Part model, mm, in its own coordinate system. A direction names the side the tool comes from. Round coordinates to 2 decimals unless told otherwise and drop trailing zeros. Loops run counter-clockwise (first coordinate to the right, second up) from the corner with the lowest first, then second, coordinate; pieces in that order, holes last. Notation, with made-up numbers: (84.25, 44) -> (134.25, 44) arc R33 cw to (134.25, 78) -> close; hole circle Ø3 at (2, -37). An arc over 180 degrees is marked (long way). Answer as CSV lines item,"result".
from build123d import *

# Parameters (mm, degrees)
SKETCH1_W           = 39
SKETCH1_H           = 39
BOSS_EXTRUDE1_DEPTH = 29
SKETCH3_W           = 37
SKETCH3_H           = 27
CUT_EXTRUDE1_DEPTH  = 38
SKETCH4_W           = 35
SKETCH4_H           = 38.588060521
CUT_EXTRUDE2_DEPTH  = 10
CUT_EXTRUDE3_START  = 27
SKETCH5_W           = 40
SKETCH5_H           = 3
CUT_EXTRUDE3_DEPTH  = 4
CUT_EXTRUDE5_START  = 38
SKETCH6_W           = 41.777462506
SKETCH6_H           = 3
CUT_EXTRUDE5_DEPTH  = 1


with BuildPart() as part:
    # Sketch1 → Boss-Extrude1 (new body)
    with BuildSketch(Plane(origin=(0, 0, 0), x_dir=(1, 0, 0), z_dir=(0, 1, 0))):
        with Locations((-4.072718242, -0.197565543)):
            Rectangle(SKETCH1_W, SKETCH1_H)
    extrude(amount=BOSS_EXTRUDE1_DEPTH)

    # Sketch3 → Cut-Extrude1 (cut)
    with BuildSketch(Plane.XY.offset(19.697565543)):
        with Locations((-4.072718242, 14.5)):
            Rectangle(SKETCH3_W, SKETCH3_H)
    extrude(amount=-CUT_EXTRUDE1_DEPTH, mode=Mode.SUBTRACT)

    # Sketch4 → Cut-Extrude2 (cut)
    with BuildSketch(Plane(origin=(0, 29, 0), x_dir=(1, 0, 0), z_dir=(0, 1, 0))):
        with Locations((-4.072718242, -0.991595804)):
            Rectangle(SKETCH4_W, SKETCH4_H)
    extrude(amount=-CUT_EXTRUDE2_DEPTH, mode=Mode.SUBTRACT)

    # Sketch5 → Cut-Extrude3 (cut)
    with BuildSketch(Plane(origin=(0, 1, 0), x_dir=(1, 0, 0), z_dir=(0, 1, 0)).offset(CUT_EXTRUDE3_START)):
        with Locations((-4.288618926, -0.197565543)):
            Rectangle(SKETCH5_W, SKETCH5_H)
    extrude(amount=CUT_EXTRUDE3_DEPTH, mode=Mode.SUBTRACT)

    # Sketch6 → Cut-Extrude5 (cut)
    with BuildSketch(Plane.XY.offset(-18.302434457).offset(CUT_EXTRUDE5_START)):
        with Locations((-4.415990597, 14.5)):
            Rectangle(SKETCH6_W, SKETCH6_H)
    extrude(amount=-CUT_EXTRUDE5_DEPTH, mode=Mode.SUBTRACT)


solid = part.part
Q1. Saw through at A-A, the plane y = 20. Write the cut outline in (x, z), then the cut area to 3 significant figures.
Geometry results:
outline,"(-23.57, -19.3) -> (15.43, -19.3) -> (15.43, 19.7) -> (14.43, 19.7) -> (14.43, -18.3) -> (-22.57, -18.3) -> (-22.57, 19.7) -> (-23.57, 19.7) -> close"
area,"115 mm2"
Q2. Saw through at B-B, the plane x = 10.5. Write the cut outline in (y, z), then the cut area to 3 significant figures.
Geometry results:
outline,"(0, -19.3) -> (29, -19.3) -> (29, -18.3) -> (1, -18.3) -> (1, 19.7) -> (0, 19.7) -> close"
area,"67.0 mm2"
Q3. Two-plate mould, pull along X, no slides. Class faces 5 (the face through (-22, 28, -10)), 6 (the face through (-23, 15, 18.698)): pulls with the +X half, pulls with the -X half, needs draft (parallel to the pull), parting line crosses it, or undercut.
Geometry results:
face 5,"undercut"
face 6,"needs draft"
Q4. Which spindle directions (+Z, -Z, +X, -X, +Y, -Y) get a long thin tool onto all of the face, cutting with end or side? Do faces 1 (the face through (-23, 29, 11)), 2 (the face through (15, 15, 18.698)), 3 (the face through (14.427, 14, 1)), 4 (the face through (15, 28, 0)). Say none if no direction does.
Geometry results:
face 1,"+Z, -Z, +X, -X, +Y"
face 2,"+Z, +X, -X"
face 3,"+Z"
face 4,"+X, -X, +Y"
Q5. Saw through at C-C, the plane z = 11. Write the cut outline in (x, y), then the cut area to 3 significant figures.
Geometry results:
outline,"(-23.57, 0) -> (15.43, 0) -> (15.43, 29) -> (13.43, 29) -> (13.43, 28) -> (14.43, 28) -> (14.43, 1) -> (-22.57, 1) -> (-22.57, 28) -> (-21.57, 28) -> (-21.57, 29) -> (-23.57, 29) -> close"
area,"97.0 mm2"
Q6. Drill centre lines: line 1 along X through (y, z) = (18, 15.5); line 2 along Z through (x, y) = (-11.5, 23.25); line 3 along Y through (x, z) = (-14.5, -12.5). Where is each one in solid material? Low to high.
Geometry results:
line 1,"-23.57 to -22.57, 14.43 to 15.43"
line 2,"-19.3 to -18.3"
line 3,"0 to 1"
Q7. Drop flat-ended pins along their axis: P1, Ø0.5, axis at x = 15, z = 0, coming from the +Y side; P2, Ø2, axis at x = -8, y = 26, coming from the +Z side; P3, Ø8, axis at x = 2.5, z = -2.5, coming from the +Y side. Give the stop position or say it passes through.
Geometry results:
P1,"y = 28"
P2,"z = -18.3"
P3,"y = 1"
